Can you work these out from the drawing? Everything is in mm from the part's minimum corner. A direction names the side the tool comes from. Round coordinates to 2 decimals unless told otherwise and drop trailing zeros. Loops run counter-clockwise (first coordinate to the right, second up) from the corner with the lowest first, then second, coordinate; pieces in that order, holes last. Notation, with made-up numbers: (70.25, -39.5) - (114.25, -39.5) arc R19 cw to (114.25, -12.5) - close; hole circle Ø7 at (-3.5, 88). An arc over 180 degrees is marked (long way). Answer as a JSON object with one key per item and string values. Group by question number.
1) Will these pins go through, and if not, where does the flat tip stop? P1, Ø1.3, axis at y = 13, z = 26, coming from the +X side (1 decimal); P2, Ø4, axis at x = 22.5, z = 7, coming from the -Y side; P3, Ø4, axis at x = 9, y = 17, coming from the -Z side; P4, Ø13, axis at x = 20, z = 12.5, coming from the +Y side.
2) Which directions (+Z, -Z, +X, -X, +Y, -Y) give clear straight access to the entire face, cutting with the end or side of a thin tool? Please do the marked faces 1 and 2.
3) I want a section at D-D, the plane y = 12.5. Please give me the cut outline in (x, z) (1 decimal).
4) If we mould it in two halves opening along Z, with no side actions, what happens to the marked faces 3, 4 and 5? For each: pulls with the +Z half, pulls with the -Z half, needs draft (parallel to the pull), parting line crosses it, or undercut.
5) If I drill on line 1 along Y through (x, z) = (2, 19.25); line 2 along Z through (x, y) = (23.5, 17.5) (1 decimal); line 3 along X through (y, z) = (10, 15), over which ranges is the centre line in solid material (lowest first)? Write a range as [from, to].
6) I want a section at C-C, the plane y = 3. Please give me the cut outline in (x, z) (1 decimal).
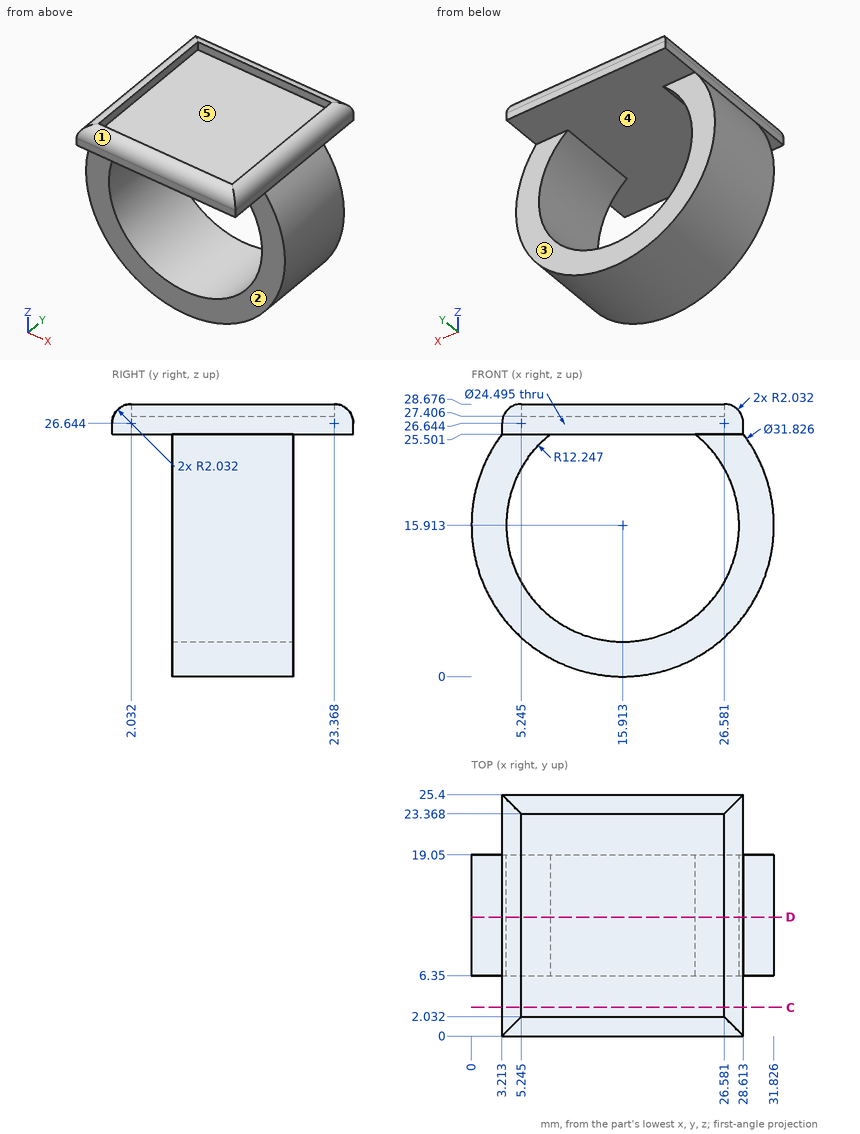
Outcome:
{
 "1": {"P1": "x = 28.7", "P2": "y = 6.35", "P3": "z = 0.78", "P4": "through"},
 "2": {"face 1": "+Z, +X, -X, -Y", "face 2": "-Z, +X, -X, -Y"},
 "3": {"outline": "(3.2, 25.5) arc R15.9 ccw (long way) to (28.6, 25.5) - (28.6, 26.6) arc R2 ccw to (26.6, 28.7) - (26.6, 27.4) - (5.2, 27.4) - (5.2, 28.7) arc R2 ccw to (3.2, 26.6) - close; hole (8.3, 25.5) arc R12.2 ccw (long way) to (23.5, 25.5) - close"},
 "4": {"face 3": "needs draft", "face 4": "undercut", "face 5": "pulls with the +Z half"},
 "5": {"line 1": "[6.35, 19.05]", "line 2": "[1.9, 6.3], [25.5, 27.4]", "line 3": "[0.03, 3.7], [28.13, 31.8]"},
 "6": {"outline": "(3.2, 25.5) - (28.6, 25.5) - (28.6, 26.6) arc R2 ccw to (26.6, 28.7) - (26.6, 27.4) - (5.2, 27.4) - (5.2, 28.7) arc R2 ccw to (3.2, 26.6) - close"}
}
